Source: CAD feature listing. Evaluate the final solid. Frame: model axes, mm. A direction names the side the tool comes from. Give positions to 0.01 mm unless a question says otherwise; leave off trailing zeros. Loops run counter-clockwise (first coordinate to the right, second up) from the corner with the lowest first, then second, coordinate; pieces in that order, holes last. Notation, with made-up numbers: M 52,32.25 L 91,32.25 A37 ccw 91,69.25 Z; hole C 43,-27 d5. An arc over 180 degrees is marked long. Answer in a Markdown table with one row per item.
```python
from build123d import *

# Parameters (mm, degrees)
BOSS_EXTRUDE1_DEPTH = 3


with BuildPart() as part:
    # Sketch2 → Boss-Extrude1 (new body)
    with BuildSketch(Plane(origin=(0, 0, 0), x_dir=(0, 0, -1), z_dir=(1, 0, 0))):
        Polygon((0, 0), (-95.762049044, 54.126056228), (-83.922091974, 81.649962502), (-86.677929554, 82.835440985), (-80.750537142, 96.614628885), (-77.994699562, 95.429150402), (-52.294504689, 155.173434164), (-55.050342269, 156.358912646), (-49.122949857, 170.138100547), (-46.367112277, 168.952622064), (-20.666917403, 228.696905826), (-23.422754983, 229.882384308), (-17.495362571, 243.661572208), (-14.739524991, 242.476093726), (-2.899567921, 270), (102.899567921, 270), (114.739524991, 242.476093726), (117.495362571, 243.661572208), (123.422754983, 229.882384308), (120.666917403, 228.696905826), (146.367112277, 168.952622064), (149.122949857, 170.138100547), (155.050342269, 156.358912646), (152.294504689, 155.173434164), (177.994699562, 95.429150402), (180.750537142, 96.614628885), (186.677929554, 82.835440985), (183.922091974, 81.649962502), (195.762049044, 54.126056228), (100, 0), (83.327078723, 117), (92, 117), (92, 120), (80, 120), (20, 120), (8, 120), (8, 117), (16.672921277, 117), align=None)
        Polygon((24.210004629, 164.434828436), (21.840147112, 149.623218958), (24.802469008, 149.149247454), (27.172326524, 163.960856933), align=None, mode=Mode.SUBTRACT)
        Polygon((36.360717046, 240.376781042), (33.990859529, 225.565171564), (36.953181425, 225.09120006), (39.323038941, 239.902809539), align=None, mode=Mode.SUBTRACT)
        Polygon((75.197530992, 149.149247454), (72.827673476, 163.960856933), (75.789995371, 164.434828436), (78.159852888, 149.623218958), align=None, mode=Mode.SUBTRACT)
        Polygon((63.046818575, 225.09120006), (66.009140471, 225.565171564), (63.639282954, 240.376781042), (60.676961059, 239.902809539), align=None, mode=Mode.SUBTRACT)
        Polygon((-52.479172452, 47.958090467), (-37.629195925, 45.841915342), (-37.2059609, 48.811910647), (-52.055937427, 50.928085772), align=None, mode=Mode.SUBTRACT)
        Polygon((137.2059609, 48.811910647), (137.629195925, 45.841915342), (152.479172452, 47.958090467), (152.055937427, 50.928085772), align=None, mode=Mode.SUBTRACT)
    extrude(amount=BOSS_EXTRUDE1_DEPTH)


solid = part.part
```
1) Set-up query: faces 5 (the flat face through (1.48, 68.08, -189.76)), 6 (the flat face through (1.479, 67.695, 89.925)), 7 (the flat face through (0, 137, -52)), 8 (the flat face through (1.48, 57.68, -91.78)). Return all of +Z, -Z, +X, -X, +Y, -Y with unobstructed straight access to the full face (end or side cutting, diameter ignored); none if empty.
Reply:
| item | result |
|---|---|
| face 5 | -Z, +X, -X |
| face 6 | +Z, +X, -X |
| face 7 | +Z, -Z, -X, +Y, -Y |
| face 8 | +X, -X, -Y |
2) Pin query (flat end, axial travel): pin 1 Ø1 at (x, z) = (2, -142.5) entering from -Y; pin 2 Ø1 at (x, z) = (1, -119) entering from -Y; pin 3 Ø1.5 at (x, y) = (2, 119) entering from +Z. Return the tip coordinate at first contact, or that it passes through.
Reply:
| item | result |
|---|---|
| pin 1 | stops at y = 23.74 |
| pin 2 | stops at y = 10.46 |
| pin 3 | stops at z = 68.18 |
3) Section D-D, the plane y = 37.5. Return loops of the section in (x, z), then the cut area to 3 significant figures.
Reply:
| item | result |
|---|---|
| outline | M 0,-166.35 L 3,-166.35 L 3,-94.66 L 0,-94.66 Z; M 0,-5.34 L 3,-5.34 L 3,66.35 L 0,66.35 Z |
| area | 430 mm² |
4) Material intervals for L1, parallel to Y at x = 1.3, z = 46.5; L2, parallel to Z at x = 2.7, y = 239; L3, parallel to Z at x = 1.1, y = 230.5, sorted ascending.
Reply:
| item | result |
|---|---|
| L1 | y = 26.28 to 47.11, 50.14 to 169.01 |
| L2 | z = -119.5 to -63.86, -60.82 to -39.18, -36.14 to 19.5 |
| L3 | z = -123.16 to -65.22, -62.18 to -37.82, -34.78 to 23.16 |
5) Pull-direction query (Z, two-part tool) for faces 1 (the flat face through (1.479, 59.319, -8.453)), 2 (the flat face through (3, 137, -52)), 3 (the flat face through (1.48, 27.44, -148.55)), 4 (the flat face through (1.479, 26.684, 47.211)); classes: released by +Z, released by -Z, zero draft, split by the parting line, or undercut.
Reply:
| item | result |
|---|---|
| face 1 | undercut |
| face 2 | zero draft |
| face 3 | released by -Z |
| face 4 | released by +Z |
6) Section B-B, the plane z = -55. Return loops of the section in (x, y).
Reply:
| item | result |
|---|---|
| outline | M 0,120 L 3,120 L 3,270 L 0,270 Z |
7) Section C-C, the plane x = 2.15. Count the separate pieces of the cut face and the enclosed holes in it, then the cut area to 3 significant figures.
Reply:
| item | result |
|---|---|
| separate pieces | 1 |
| enclosed holes | 6 |
| area | 43,500 mm² |
8) Section A-A, the plane y = 75. Return loops of the section in (x, z).
Reply:
| item | result |
|---|---|
| outline | M 0,-186.78 L 3,-186.78 L 3,-89.31 L 0,-89.31 Z; M 0,-10.69 L 3,-10.69 L 3,86.78 L 0,86.78 Z |
